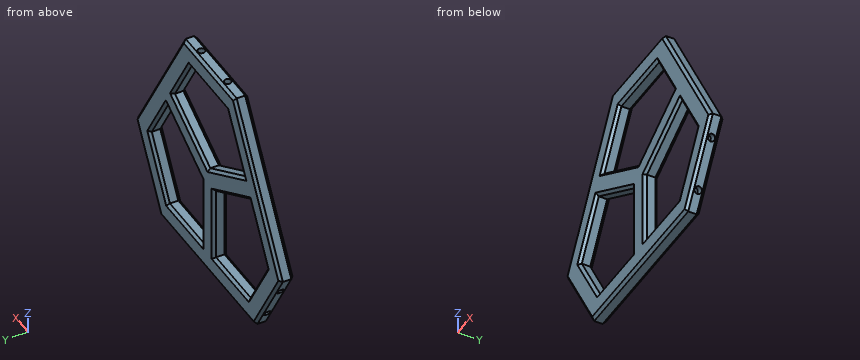
from build123d import *

# Parameters (mm, degrees)
BOSS_EXTRUDE1_DEPTH        = 5
BOSS_EXTRUDE1_DEPTH_BACK   = 5
M3X6X5_INSERT_HOLES1_D     = 5
M3X6X5_INSERT_HOLES1_DEPTH = 6.5
M3X6X5_INSERT_HOLES2_D     = 5
M3X6X5_INSERT_HOLES2_DEPTH = 6.5
M3X6X5_INSERT_HOLES3_D     = 5
M3X6X5_INSERT_HOLES3_DEPTH = 6.5
CUT_EXTRUDE3_DEPTH         = 132.434394281
CHAMFER3_SIZE              = 2


with BuildPart() as part:
    # Sketch1 → Boss-Extrude1 (new, two sides: drawn at the far end of the back side and taken through both)
    with BuildSketch(Plane(origin=(0, 0, 0), x_dir=(1, 0, 0), z_dir=(0, 1, 0)).offset(-BOSS_EXTRUDE1_DEPTH_BACK)):
        Polygon((-61.782032303, 72.990381057), (-95.262794416, 15), (-34.641016151, -90), (32.320508076, -90), (94.102540378, 17.009618943), (61.782032303, 72.990381057), align=None)
    extrude(amount=BOSS_EXTRUDE1_DEPTH + BOSS_EXTRUDE1_DEPTH_BACK)

    # M3x6x5 Insert Holes1
    with Locations(Plane.XY.offset(90)):
        with Locations((-17.320508076, 0), (17.320508076, 0)):
            Hole(M3X6X5_INSERT_HOLES1_D / 2, depth=M3X6X5_INSERT_HOLES1_DEPTH)

    # M3x6x5 Insert Holes2
    with Locations(Plane(origin=(77.942286341, 0, -45), x_dir=(-0.5000000000000001, 0, -0.8660254037844386), z_dir=(0.8660254037844386, 0, -0.5000000000000001))):
        with Locations((-17.320508076, 0), (17.320508076, 0)):
            Hole(M3X6X5_INSERT_HOLES2_D / 2, depth=M3X6X5_INSERT_HOLES2_DEPTH)

    # M3x6x5 Insert Holes3
    with Locations(Plane(origin=(-77.942286341, 0, -45), x_dir=(-0.5000000000000003, 0, 0.8660254037844386), z_dir=(-0.8660254037844386, 0, -0.5000000000000003))):
        with Locations((-17.320508076, 0), (17.320508076, 0)):
            Hole(M3X6X5_INSERT_HOLES3_D / 2, depth=M3X6X5_INSERT_HOLES3_DEPTH)

    # Sketch10 → Cut-Extrude3 (cut, through all)
    with BuildSketch(Plane(origin=(0, 5, 0), x_dir=(1, 0, 0), z_dir=(0, 1, 0))):
        Polygon((-7.5, 57.990381057), (-53.121778265, 57.990381057), (-77.942286341, 15), (-55.711524227, -23.504809472), (-7.5, 4.330127019), align=None)
        Polygon((7.5, 57.990381057), (53.121778265, 57.990381057), (76.782032303, 17.009618943), (53.97114317, -22.5), (7.5, 4.330127019), align=None)
        Polygon((46.47114317, -35.490381057), (23.660254038, -75), (-25.980762114, -75), (-48.211524227, -36.495190528), (0, -8.660254038), align=None)
    extrude(amount=-CUT_EXTRUDE3_DEPTH, mode=Mode.SUBTRACT)

    # Chamfer3
    chamfer3_edges = [part.edges().sort_by_distance(p)[0] for p in [
        (-64.951905284, -5, 37.5),
        (-1.160254038, -5, 90),
        (0, 5, -72.990381057),
        (-78.52241336, 5, -43.995190528),
        (-64.951905284, 5, 37.5),
        (-1.160254038, 5, 90),
        (63.211524227, 5, 36.495190528),
        (77.942286341, 5, -45),
        (63.211524227, -5, 36.495190528),
        (77.942286341, -5, -45),
        (0, -5, -72.990381057),
        (23.235571585, -5, 22.075317547),
        (35.065698604, -5, 55.245190528),
        (-1.160254038, -5, 75),
        (-37.09614317, -5, 55.747595264),
        (-24.105762114, -5, 22.577722283),
        (23.235571585, 5, 22.075317547),
        (-24.105762114, 5, 22.577722283),
        (-37.09614317, 5, 55.747595264),
        (-1.160254038, 5, 75),
        (35.065698604, 5, 55.245190528),
        (-65.532032303, -5, -36.495190528),
        (-30.310889132, -5, -57.990381057),
        (-7.5, -5, -31.160254038),
        (-31.605762114, -5, 9.587341226),
        (-66.826905284, -5, 4.252404736),
        (-65.532032303, 5, -36.495190528),
        (-66.826905284, 5, 4.252404736),
        (-31.605762114, 5, 9.587341226),
        (-7.5, 5, -31.160254038),
        (-30.310889132, 5, -57.990381057),
        (7.5, -5, -31.160254038),
        (30.310889132, -5, -57.990381057),
        (64.951905284, -5, -37.5),
        (65.376587737, -5, 2.745190528),
        (30.735571585, -5, 9.084936491),
        (7.5, 5, -31.160254038),
        (30.735571585, 5, 9.084936491),
        (65.376587737, 5, 2.745190528),
        (64.951905284, 5, -37.5),
        (30.310889132, 5, -57.990381057),
        (-78.52241336, -5, -43.995190528),
    ]]
    chamfer(chamfer3_edges, length=CHAMFER3_SIZE)


solid = part.part
Input: part model. Units: mm. Frame: model coordinates. Round coordinates to 2 decimals unless told otherwise and drop trailing zeros. Loops run counter-clockwise (first coordinate to the right, second up) from the corner with the lowest first, then second, coordinate; pieces in that order, holes last. Notation, with made-up numbers: (24, 22) -> (69, 22) arc R17 cw to (69, 35) -> close; hole circle Ø3 at (-24.5, 38.25). An arc over 180 degrees is marked (long way). Answer as a JSON object with one key per item and string values. Group by question number.
1) Section query B-B on x = -42. Output: boundary loops of the cut face in (y, z).
2) Section query D-D on x = -73.5. Output: boundary loops of the cut face in (y, z), plus the area to 3 significant figures.
3) Ray query, L1, parallel to Z at x = -24.5, y = -2; L2, parallel to X at y = -0.25, z = 9; L3, parallel to Z at x = 27, y = -2. Return the intervals inside material, ascending.
4) Section query C-C on z = 63.5. Output: boundary loops of the cut face in (x, y).
5) Section query A-A on z = 20. State how many separate pieces and enclosed holes the cut face has, plus the area to 3 significant figures.
6) Pin query (flat end, axial travel): pin 1 (1 mm diameter, centred on y = 0, z = -13, fed in from +X); pin 2 (4 mm diameter, centred on x = -17.32, y = 0, fed in from +Z); pin 3 (1.8 mm diameter, centred on y = -1, z = -20.5, fed in from -X). Return the tip coordinate at first contact, or that it passes through.
Reply:
{
 "1": {"outline": "(-5, -70.99) -> (-3, -72.99) -> (3, -72.99) -> (5, -70.99) -> (5, -59.99) -> (3, -57.99) -> (-3, -57.99) -> (-5, -59.99) -> close; (-5, 17.9) -> (-3, 15.59) -> (3, 15.59) -> (5, 17.9) -> (5, 30.6) -> (3, 32.91) -> (-3, 32.91) -> (-5, 30.6) -> close; (-5, 51.25) -> (-3, 47.25) -> (3, 47.25) -> (5, 51.25) -> (5, 73.25) -> (3, 77.25) -> (-3, 77.25) -> (-5, 73.25) -> close"},
 "2": {"outline": "(-5, -48.69) -> (-3, -52.69) -> (3, -52.69) -> (5, -48.69) -> (5, -26.69) -> (3, -22.69) -> (-3, -22.69) -> (-5, -26.69) -> close; (-5, -3.31) -> (-3, -7.31) -> (3, -7.31) -> (5, -3.31) -> (5, 18.69) -> (3, 22.69) -> (-3, 22.69) -> (-5, 18.69) -> close", "area": "568 mm2"},
 "3": {"L1": "z = -72.99 to -57.99, 5.48 to 22.81, 75 to 90", "L2": "x = -81.41 to -64.09, -30.59 to -0.59, 0.59 to 30.59, 61.77 to 79.09", "L3": "z = -72.99 to -57.99, 6.93 to 24.25, 69.22 to 90"},
 "4": {"outline": "(-49.94, -3) -> (-47.63, -5) -> (-34.93, -5) -> (-32.62, -3) -> (-32.62, 3) -> (-34.93, 5) -> (-47.63, 5) -> (-49.94, 3) -> close; (30.3, -3) -> (32.61, -5) -> (45.31, -5) -> (47.62, -3) -> (47.62, 3) -> (45.31, 5) -> (32.61, 5) -> (30.3, 3) -> close"},
 "5": {"separate pieces": "4", "enclosed holes": "0", "area": "896 mm2"},
 "6": {"pin 1": "stops at x = 92.08", "pin 2": "stops at z = 83.5", "pin 3": "stops at x = -92.61"}
}
